```python
from build123d import *

# Parameters (mm, degrees)
BOSS_EXTRUDE1_DEPTH = 3


with BuildPart() as part:
    # Sketch1 → Boss-Extrude1 (new body)
    with BuildSketch(Plane.XY):
        Polygon((0, 60), (0, 50), (-3, 50), (-3, 40), (0, 40), (0, 30), (-3, 30), (-3, 20), (0, 20), (0, 10), (-3, 10), (-3, 0), (-3, -3), (0, -3), (10, -3), (10, 0), (20, 0), (20, -3), (30, -3), (30, 0), (40, 0), (40, -3), (50, -3), (50, 0), (60, 0), (60, -3), (70, -3), (70, 0), (80, 0), (80, -3), (90, -3), (90, 0), (100, 0), (100, -3), (110, -3), (110, 0), (120, 0), (120, -3), (130, -3), (130, 0), (140, 0), (140, -3), (150, -3), (153, -3), (153, 0), (153, 10), (150, 10), (150, 20), (153, 20), (153, 30), (150, 30), (150, 40), (153, 40), (153, 50), (150, 50), (150, 60), (153, 60), (153, 70), (153, 73), (150, 73), (140, 73), (140, 70), (130, 70), (130, 73), (120, 73), (120, 70), (110, 70), (110, 73), (100, 73), (100, 70), (90, 70), (90, 73), (80, 73), (80, 70), (70, 70), (70, 73), (60, 73), (60, 70), (50, 70), (50, 73), (40, 73), (40, 70), (30, 70), (30, 73), (20, 73), (20, 70), (10, 70), (10, 73), (0, 73), (-3, 73), (-3, 70), (-3, 60), align=None)
    extrude(amount=BOSS_EXTRUDE1_DEPTH)


solid = part.part
```
Read the model definition and answer for the solid it produces. Units are mm, in the model's axes. A direction names the side the tool comes from. Coordinates: 2 decimals unless noted, no trailing zeros. Write each loop counter-clockwise with the first axis right and the second up, starting at its lowest first coordinate (ties: lowest second). Pieces come first, ordered by that corner, then holes. Notation, with made-up numbers: (27, -23.5) - (48, -23.5) arc R20 cw to (48, -17.5) - close; hole circle Ø8 at (-30, 58). An arc over 180 degrees is marked (long way). Answer as a JSON object with one key per item and string values. Group by question number.
1. A cutting plane is placed at A-A (x = 78.5). Determine the outline of the cut face in (y, z), plus the area to 3 significant figures.
2. The mould has two halves that part along Y. Classify faces 1 (the flat face through (10, -2, 1)), 2 (the flat face through (150, 55, 1)), 3 (the flat face through (125, 73, 1)), 4 (the flat face through (135, 0, 1)): +Y half, -Y half, draft (parallel to the pull), parting line (faces both ways), or undercut.
3. Which of the six approach directions +Z, -Z, +X, -X, +Y, -Y give full straight-line access (tool end or side, diameter ignored) to faces 5 (the flat face through (0, 15, 1)), 6 (the flat face through (75, 0, 1)), 7 (the flat face through (65, 73, 1)), 8 (the flat face through (20, 72, 1))?
4. This flat-tipped pin is pushed along its axis until it touches: P1, Ø0.9, axis at x = 75.5, z = 1, coming from the +Y side. Where does it stop, or does it pass through?
5. Consider L1, parallel to Y at x = 53.5, z = 0.6; L2, parallel to X at y = 51, z = 2.55. Determine where each line is inside the solid, lowest interval first. Write a range as [from, to].
Worked out:
{
 "1": {"outline": "(0, 0) - (70, 0) - (70, 3) - (0, 3) - close", "area": "210 mm²"},
 "2": {"face 1": "draft", "face 2": "undercut", "face 3": "+Y half", "face 4": "-Y half"},
 "3": {"face 5": "+Z, -Z, -X", "face 6": "+Z, -Z, -Y", "face 7": "+Z, -Z, +X, -X, +Y", "face 8": "+Z, -Z, +Y"},
 "4": {"P1": "stops at y = 70"},
 "5": {"L1": "y = [0, 70]", "L2": "x = [0, 150]"}
}
